Design review of the part built by this model. Coordinates are the model's own, in mm. Face numbers are marked on the shaded views. Coordinates: 2 decimals unless noted, no trailing zeros. Loops run counter-clockwise (first coordinate to the right, second up) from the corner with the lowest first, then second, coordinate; pieces in that order, holes last. Notation, with made-up numbers: (6, 19.5) -> (50, 19.5) arc R17 ccw to (50, 27.5) -> close; hole circle Ø1 at (6.25, 62.5). An arc over 180 degrees is marked (long way). Answer as a JSON object with one key per item and string values.
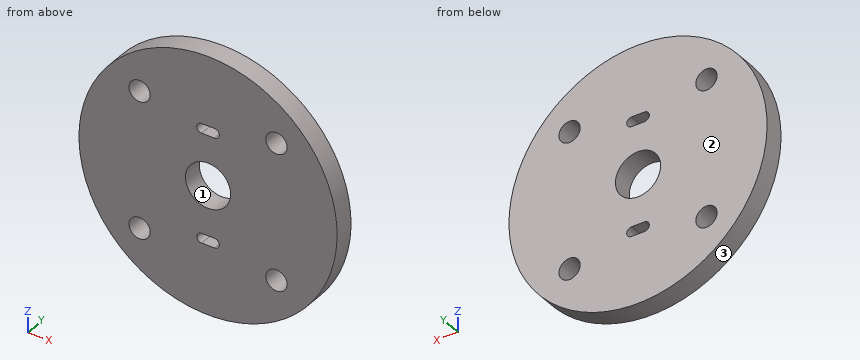
```python
from build123d import *

# Parameters (mm, degrees)
SKETCH1_R           = 20
SKETCH1_R_2         = 3.5
SKETCH1_R_3         = 1.65
BOSS_EXTRUDE1_DEPTH = 3.175
CUT_EXTRUDE1_DEPTH  = 44.400561775


with BuildPart() as part:
    # Sketch1 → Boss-Extrude1 (new body)
    with BuildSketch(Plane(origin=(0, 0, 0), x_dir=(1, 0, 0), z_dir=(0, 1, 0))):
        with Locations(Location((10.606601718, 10.606601718, 0), (0, 0, 270))):
            Circle(SKETCH1_R)
        with Locations(Location((10.606601718, 10.606601718, 0), (0, 0, 270))):
            Circle(SKETCH1_R_2, mode=Mode.SUBTRACT)
        with Locations(Location((0, 21.213203436, 0), (0, 0, 270))):
            Circle(SKETCH1_R_3, mode=Mode.SUBTRACT)
        with Locations(Location((21.213203436, 21.213203436, 0), (0, 0, 270))):
            Circle(SKETCH1_R_3, mode=Mode.SUBTRACT)
        with Locations(Location((21.213203436, 0, 0), (0, 0, 270))):
            Circle(SKETCH1_R_3, mode=Mode.SUBTRACT)
        with Locations(Location((0, 0, 0), (0, 0, 270))):
            Circle(SKETCH1_R_3, mode=Mode.SUBTRACT)
    extrude(amount=BOSS_EXTRUDE1_DEPTH)

    # Sketch2 → Cut-Extrude1 (cut, through all)
    with BuildSketch(Plane(origin=(0, 3.175, 0), x_dir=(1, 0, 0), z_dir=(0, 1, 0))):
        with BuildLine():
            Line((9.606601718, 19.856601736), (11.606601718, 19.856601736))
            ThreePointArc((11.606601718, 19.856601736), (12.356601718, 19.106601736), (11.606601718, 18.356601736))
            Line((11.606601718, 18.356601736), (9.606601718, 18.356601736))
            ThreePointArc((9.606601718, 18.356601736), (8.856601718, 19.106601736), (9.606601718, 19.856601736))
        make_face()
        with BuildLine():
            Line((9.606601718, 1.3566017), (11.606601718, 1.3566017))
            ThreePointArc((11.606601718, 1.3566017), (12.356601718, 2.1066017), (11.606601718, 2.8566017))
            Line((11.606601718, 2.8566017), (9.606601718, 2.8566017))
            ThreePointArc((9.606601718, 2.8566017), (8.856601718, 2.1066017), (9.606601718, 1.3566017))
        make_face()
    extrude(amount=-CUT_EXTRUDE1_DEPTH, mode=Mode.SUBTRACT)


solid = part.part
```
1) Add section B-B, the plane z = -8.5. Give the boundary of the cut face in (x, y) (3 decimals), and give its area (3 significant figures).
Completed:
{"outline": "(-9.282, 0) -> (7.812, 0) -> (7.812, 3.175) -> (-9.282, 3.175) -> close; (13.402, 0) -> (30.495, 0) -> (30.495, 3.175) -> (13.402, 3.175) -> close", "area": "109 mm²"}
2) Wall thickness on probe 1 along X at (y, z) = (3, -1.5); probe 2 along X at (y, z) = (1.8, -21.5); probe 3 along X at (y, z) = (2.3, -13): over which ranges is each line inside the solid? List them lowest first.
Completed:
{"probe 1": "-7.2 to -0.69, 0.69 to 9.17, 12.05 to 20.53, 21.9 to 28.41", "probe 2": "-6.17 to -1.62, 1.62 to 19.59, 22.84 to 27.38", "probe 3": "-9.25 to 8.05, 13.16 to 30.46"}
3) Clearance check with a flat-ended pin moving along its axis: pin 1 Ø1 at (x, y) = (11, 2.5) entering from +Z. State where the tip first meets the part, or that it passes through.
Completed:
{"pin 1": "z = 9.39"}
4) Add section A-A, the plane z = 0. Give the boundary of the cut face in (x, y) (3 decimals), and give its area (3 significant figures).
Completed:
{"outline": "(-6.349, 0) -> (-1.65, 0) -> (-1.65, 3.175) -> (-6.349, 3.175) -> close; (1.65, 0) -> (19.563, 0) -> (19.563, 3.175) -> (1.65, 3.175) -> close; (22.863, 0) -> (27.562, 0) -> (27.562, 3.175) -> (22.863, 3.175) -> close", "area": "86.7 mm²"}
5) The part is to be moulded in two halves that separate along X. For the marked faces 1, 2 and 3, say which applies: pulls with the +X half, pulls with the -X half, needs draft (parallel to the pull), parting line crosses it, or undercut.
Completed:
{"face 1": "undercut", "face 2": "needs draft", "face 3": "parting line crosses it"}
6) Add section D-D, the plane y = 1.8. Give the boundary of the cut face in (x, z), and give its area (3 significant figures).
Completed:
{"outline": "circle Ø40 at (10.61, -10.61); hole circle Ø3.3 at (0, -21.21); hole circle Ø3.3 at (0, 0); hole circle Ø7 at (10.61, -10.61); hole (9.61, -19.86) -> (11.61, -19.86) arc R0.75 ccw to (11.61, -18.36) -> (9.61, -18.36) arc R0.75 ccw to start; hole (9.61, -2.86) -> (11.61, -2.86) arc R0.75 ccw to (11.61, -1.36) -> (9.61, -1.36) arc R0.75 ccw to start; hole circle Ø3.3 at (21.21, -21.21); hole circle Ø3.3 at (21.21, 0)", "area": "1,170 mm²"}
7) Add section C-C, the plane x = 0. Give the boundary of the cut face in (y, z) (3 decimals), and give its area (3 significant figures).
Completed:
{"outline": "(0, -27.562) -> (3.175, -27.562) -> (3.175, -22.863) -> (0, -22.863) -> close; (0, -19.563) -> (3.175, -19.563) -> (3.175, -1.65) -> (0, -1.65) -> close; (0, 1.65) -> (3.175, 1.65) -> (3.175, 6.349) -> (0, 6.349) -> close", "area": "86.7 mm²"}
